Verification items for the finished model (mm, model axes). A direction names the side the tool comes from. Coordinates: 2 decimals unless noted, no trailing zeros. Loops run counter-clockwise (first coordinate to the right, second up) from the corner with the lowest first, then second, coordinate; pieces in that order, holes last. Notation, with made-up numbers: M 47,-35 L 58,-35 A20 ccw 58,-23 Z; hole C -4,18 d3. An arc over 180 degrees is marked long. Write item = value, one per line. Start each with the question number.
```python
from build123d import *

# Parameters (mm, degrees)
F0_R          = 6.5
F1_DEPTH      = 3.5
F1_DEPTH_BACK = 3.5
F2_R          = 9
F3_DEPTH      = 0.75
F4_R          = 9
F5_DEPTH      = 0.75
F6_R          = 2
F7_DEPTH      = 25
F7_DEPTH_BACK = 25


with BuildPart() as f1:
    # F0 (on Right) → F1 (new body, two sides)
    with BuildSketch(Plane.YZ) as f1_sk:
        Circle(F0_R)
    extrude(amount=F1_DEPTH)
    extrude(f1_sk.sketch, amount=-F1_DEPTH_BACK)

    # F2 (on face) → F3 (join)
    with BuildSketch(Plane.YZ.offset(3.5)):
        Circle(F2_R)
    extrude(amount=F3_DEPTH)

    # F4 (on face) → F5 (join)
    with BuildSketch(Plane(origin=(-3.5, 0, 0), x_dir=(0, -1, 0), z_dir=(-1, 0, 0))):
        Circle(F4_R)
    extrude(amount=F5_DEPTH)

    # F6 (on Right) → F7 (cut, two sides)
    with BuildSketch(Plane.YZ) as f7_sk:
        Circle(F6_R)
    extrude(amount=-F7_DEPTH, mode=Mode.SUBTRACT)
    extrude(f7_sk.sketch, amount=F7_DEPTH_BACK, mode=Mode.SUBTRACT)


solid = f1.part
```
Q1. Sectioned sample at A-A on z = 0. Record the cut outline in (x, y).
Q2. Set-up check for faces 4 (the face through (0.049, -5.158, -3.955)), 5 (the face through (-3.87, 1.172, 8.923)): record each of +Z, -Z, +X, -X, +Y, -Y from which the full face is reachable in a straight line by a thin tool's end or side.
Q3. Scan lines: L1, parallel to Z at x = -1, y = 0; L2, parallel to X at y = -7.5, z = 1.25; L3, parallel to Z at x = 1.5, y = -1.25. Record each from-to range of solid material in increasing order. Write a range as [from, to].
Q4. Gauge pin test, flat ends, axial feed: pin 1 (2 mm diameter, centred on x = 1, y = 1, fed in from +Z); pin 2 (1.5 mm diameter, centred on x = -1, z = -6.5, fed in from +Y). Record the tip position at first contact, or that the pin passes through.
Q5. Sectioned sample at D-D on y = -8. Record the cut outline in (x, z), plus the area to 3 significant figures.
Q6. Mould release check, pull along X, two halves, no side actions. Record for faces 1 (the face through (3.5, 3, -6)), 2 (the face through (-4.25, -2, -2)), 3 (the face through (4.25, 2, -2)): +X half, -X half, draft (parallel to the pull), parting line (faces both ways), or undercut.
Q7. Sectioned sample at C-C on x = 2.75. Record the cut outline in (y, z), plus the area to 3 significant figures.
Solutions:
q1.outline = M -4.25,-9 L -3.5,-9 L -3.5,-6.5 L 3.5,-6.5 L 3.5,-9 L 4.25,-9 L 4.25,-2 L -4.25,-2 Z; M -4.25,2 L 4.25,2 L 4.25,9 L 3.5,9 L 3.5,6.5 L -3.5,6.5 L -3.5,9 L -4.25,9 Z
q2.face_4 = none
q2.face_5 = +X, -X
q3.L1 = [-6.5, -2], [2, 6.5]
q3.L2 = [-4.25, -3.5], [3.5, 4.25]
q3.L3 = [-6.38, -1.56], [1.56, 6.38]
q4.pin_1 = 6.5
q4.pin_2 = 3.03
q5.outline = M -4.25,-4.12 L -3.5,-4.12 L -3.5,4.12 L -4.25,4.12 Z; M 3.5,-4.12 L 4.25,-4.12 L 4.25,4.12 L 3.5,4.12 Z
q5.area = 12.4 mm²
q6.face_1 = undercut
q6.face_2 = -X half
q6.face_3 = +X half
q7.outline = C 0,0 d13; hole C 0,0 d4
q7.area = 120 mm²
